Autodesk Fusion 360 part; units mm, degrees
sketch "Sketch1" plane through (0, 0, 0) normal (0, 1, 0) x (1, 0, 0)
  line L0 (-3.75, 19.5) -> (3.75, 19.5)
  line L1 (3.75, 19.5) -> (3.75, -19.5)
  line L2 (3.75, -19.5) -> (-3.75, -19.5)
  line L3 (-3.75, -19.5) -> (-3.75, 19.5)
  line L4 (-3.75, 19.5) -> (3.75, -19.5) construction
  line L5 (3.75, 19.5) -> (-3.75, -19.5) construction
  circle A0 centre (-66.05, 0) radius 15
  line L6 (-3.75, -19.5) -> (-67.1215, -14.9617)
  line L7 (-3.75, 19.5) -> (-67.1215, 14.9617)
  dimension "d1" = 7.5
  dimension "d2" = 39
  dimension "d4" = 30
extrude "Extrude1" add sketch "Sketch1" along normal blind 6
sketch "Sketch2" plane through (0, 6, 0) normal (0, 1, 0) x (-1, 0, 0)
  line L0 (-3.75, -19.5) -> (3.75, -19.5)
  line L1 (3.75, -19.5) -> (67.1215, -14.9617)
  arc A0 (67.1215, -14.9617) -> (67.1215, 14.9617) centre (66.05, 0) ccw
  line L2 (67.1215, 14.9617) -> (3.75, 19.5)
  line L3 (3.75, 19.5) -> (-3.75, 19.5)
  line L4 (-3.75, 19.5) -> (-3.75, -19.5)
  line L5 (-3.75, 19.5) -> (3.75, 19.5)
  line L6 (3.75, 19.5) -> (3.75, -19.5)
  line L7 (3.75, -19.5) -> (-3.75, -19.5)
  line L8 (-3.75, -19.5) -> (-3.75, 19.5)
  line L9 (-3.75, 19.5) -> (3.75, -19.5) construction
  line L10 (3.75, 19.5) -> (-3.75, -19.5) construction
  dimension "d7" = 7.5
  dimension "d8" = 39
extrude "Extrude2" add sketch "Sketch2" against normal blind 20.2 contours L0 L3 L4 L5 L6 L7 L8
sketch "Sketch3" plane through (0, 6, 0) normal (0, 1, 0) x (-1, 0, 0)
  line L0 (3.75, -19.5) -> (67.1215, -14.9617)
  arc A0 (67.1215, -14.9617) -> (67.1215, 14.9617) centre (66.05, 0) ccw
  line L1 (67.1215, 14.9617) -> (3.75, 19.5)
  line L2 (3.75, 19.5) -> (-3.75, 19.5)
  line L3 (-3.75, 19.5) -> (-3.75, -19.5)
  line L4 (-3.75, -19.5) -> (3.75, -19.5)
  circle A1 centre (66.05, 0) radius 4
  dimension "d11" = 8
extrude "Extrude3" add sketch "Sketch3" against normal blind 9 contours A1
sketch "Sketch4" plane through (0, -3, 0) normal (0, -1, 0) x (1, 0, 0)
  circle A0 centre (-66.05, 0) radius 4
  circle A1 centre (-66.05, 0) radius 3
  dimension "d14" = 6
extrude "Extrude4" add sketch "Sketch4" along normal blind 6 contours A1
sketch "Sketch5" plane through (0, 6, 0) normal (0, 1, 0) x (-1, 0, 0)
  line L0 (3.75, -19.5) -> (67.1215, -14.9617)
  arc A0 (67.1215, -14.9617) -> (67.1215, 14.9617) centre (66.05, 0) ccw
  line L1 (67.1215, 14.9617) -> (3.75, 19.5)
  line L2 (3.75, 19.5) -> (-3.75, 19.5)
  line L3 (-3.75, 19.5) -> (-3.75, -19.5)
  line L4 (-3.75, -19.5) -> (3.75, -19.5)
  line L5 (3.75, -19.5) -> (23.6989, -18.0714)
  line L6 (3.75, 19.5) -> (23.6989, 18.0714)
  line L7 (23.6989, 18.0714) -> (23.6989, -18.0714)
  line L8 (23.6989, -18.0714) -> (17.7142, -18.5)
  line L9 (23.6989, 18.0714) -> (17.7142, 18.5)
  line L10 (17.7142, 18.5) -> (17.7142, -18.5)
  line L11 (17.7142, -18.5) -> (23.6989, 18.0714)
  line L12 (23.6989, -18.0714) -> (17.7142, 18.5)
  line L13 (17.7142, 0) -> (23.6989, 0)
  circle A1 centre (20.7416, 0) radius 1.6
  line L14 (20.7416, 0) -> (20.7416, 10)
  circle A2 centre (20.7416, 10) radius 1.6
  line L15 (20.7416, 0) -> (20.7416, -10)
  circle A3 centre (20.7416, -10) radius 1.6
  dimension "d17" = 20
  dimension "d18" = 20
  dimension "d19" = 6
  dimension "d20" = 6
  dimension "d21" = 3.2
  dimension "d22" = 10
  dimension "d23" = 3.2
  dimension "d24" = 10
  dimension "d25" = 3.2
extrude "Extrude5" cut sketch "Sketch5" against normal blind 13 contours A3 | L11 L13 A1 | L11 A1 L15 | L12 A1 L15 | L12 L13 A1 | A2 | L12 L13 A1 | L11 A1 L14 | L11 L13 A1 | L12 A1 L14
sketch "Sketch6" plane through (0, 0, 19.5) normal (0, 0, 1) x (1, 0, 0)
  line L0 (3.75, -14.2) -> (3.75, 6)
  line L1 (3.75, 6) -> (-3.75, 6)
  line L2 (-3.75, 6) -> (-3.75, 0)
  line L3 (-3.75, 0) -> (-3.75, -14.2)
  line L4 (-3.75, -14.2) -> (3.75, -14.2)
  line L5 (3.75, -14.2) -> (3.75, -17.07)
  line L6 (3.75, -17.07) -> (-3.75, -14.2)
  dimension "d28" = 2.87
extrude "Extrude6" add sketch "Sketch6" against normal blind 39 contours L4 L5 L6
sketch "Sketch7" plane through (-3.75, 0, 0) normal (-1, 0, 0) x (0, 0, 1)
  line L0 (19.5, 0) -> (-19.5, 0)
  line L1 (-19.5, 0) -> (-19.5, -14.2)
  line L2 (-19.5, -14.2) -> (19.5, -14.2)
  line L3 (19.5, -14.2) -> (19.5, 0)
  line L4 (-19.5, -14.2) -> (-10, -14.2)
  line L5 (-10, -14.2) -> (-10, -8.1)
  line L6 (-10, -8.1) -> (10, -8.1)
  circle A0 centre (-10, -8.1) radius 1.6
  circle A1 centre (10, -8.1) radius 1.6
  dimension "d31" = 9.5
  dimension "d32" = 6.1
  dimension "d33" = 20
  dimension "d34" = 3.2
  dimension "d35" = 3.2
extrude "Extrude7" cut sketch "Sketch7" against normal blind 61 contours A1 | L5 L6 A0 | L5 L6 A0
Part model, mm, in its own coordinate system. A direction names the side the tool comes from. Coordinates: 2 decimals unless noted, no trailing zeros. Loops run counter-clockwise (first coordinate to the right, second up) from the corner with the lowest first, then second, coordinate; pieces in that order, holes last. Notation, with made-up numbers: M 12.5,86.5 L 65.5,86.5 A21 cw 65.5,91.5 Z; hole C 12,3.25 d10. An arc over 180 degrees is marked long. Use a Markdown table: item, result. Add a question column.
Q1. Cut at D-D (y = 1.5). Write the cut outline in (x, z), and give its area (3 significant figures).
Q2. Pin check, flat tips, straight feed: P1, Ø10, axis at x = -62.5, y = -10.5, coming from the -Z side; P2, Ø2, axis at y = -14.5, z = 0, coming from the -X side; P3, Ø8, axis at x = -61.5, z = -0.5, coming from the -Y side; P4, Ø3, axis at x = -20.74, z = -10, coming from the -Y side. Stop position of each tip, or through.
Q3. Mould opens along X. For faces 3 (the cylindrical face through (-69.047, -5.958, -0.132)), 4 (the flat face through (0.052, -15.655, 0.273)), 5 (the flat face through (-66, -9, 0)), 6 (the cylindrical face through (-62.054, -1.479, 0.176)) say: +X half, -X half, draft (parallel to the pull), parting line (faces both ways), or undercut.
Q4. Cut at B-B (y = -2). Write the cut outline in (x, z).
Q5. Cut at A-A (z = 0). Write the cut outline in (x, y), and give its area (3 significant figures).
Q6. Probe L1, parallel to Y at x = -75, z = 0.5; L2, parallel to X at y = 1.9, z = 10; L3, parallel to Y at x = -1, z = -10. List the from-to ranges inside material, lowest first.
Q7. Which spindle directions (+Z, -Z, +X, -X, +Y, -Y) get a long thin tool onto all of the face, cutting with end or side? Do faces 1 (the flat face through (-38, 6, 0)), 2 (the flat face through (-68, -3, 3)). Say none if no direction does.
Q8. Cut at C-C (z = 10). Write the cut outline in (x, y).
Worked out:
| question | item | result |
|---|---|---|
| 1 | outline | M -67.12,-14.96 L -3.75,-19.5 L 3.75,-19.5 L 3.75,19.5 L -3.75,19.5 L -67.12,14.96 A15 ccw Z; hole C -20.74,-10 d3.2; hole C -20.74,0 d3.2; hole C -20.74,10 d3.2 |
| 1 | area | 2,770 mm2 |
| 2 | P1 | stops at z = -3 |
| 2 | P2 | stops at x = -3.75 |
| 2 | P3 | stops at y = -9 |
| 2 | P4 | passes through |
| 3 | face 3 | undercut |
| 3 | face 4 | -X half |
| 3 | face 5 | draft |
| 3 | face 6 | undercut |
| 4 | outline | C -66.05,0 d8; M -3.75,-19.5 L 3.75,-19.5 L 3.75,19.5 L -3.75,19.5 Z |
| 5 | outline | M -81.05,0 L -70.05,0 L -70.05,-3 L -69.05,-3 L -69.05,-9 L -63.05,-9 L -63.05,-3 L -62.05,-3 L -62.05,0 L -22.34,0 L -22.34,6 L -81.05,6 Z; M -19.14,0 L -3.75,0 L -3.75,-14.2 L 3.75,-17.07 L 3.75,6 L -19.14,6 Z |
| 5 | area | 667 mm2 |
| 6 | L1 | y = 0 to 6 |
| 6 | L2 | x = -77.23 to -22.34, -19.14 to 3.75 |
| 6 | L3 | y = -15.25 to -9.7, -6.5 to 6 |
| 7 | face 1 | +Z, -Z, +X, -X, +Y |
| 7 | face 2 | -Y |
| 8 | outline | M -77.23,0 L -22.34,0 L -22.34,6 L -77.23,6 Z; M -19.14,0 L -3.75,0 L -3.75,-6.5 L 3.75,-6.5 L 3.75,6 L -19.14,6 Z; M -3.75,-14.2 L 3.75,-17.07 L 3.75,-9.7 L -3.75,-9.7 Z |
